Source: three-view drawing plus pictorial views. Frame: mm from the lowest corner of the part. Round coordinates to 2 decimals unless told otherwise and drop trailing zeros. Write each loop counter-clockwise with the first axis right and the second up, starting at its lowest first coordinate (ties: lowest second). Pieces come first, ordered by that corner, then holes. Notation, with made-up numbers: (2.25, 0.5) - (25.25, 0.5) arc R13 ccw to (25.25, 5.5) - close; hole circle Ø10 at (35.25, 76). An arc over 180 degrees is marked (long way). Write each question's results on one line, items separated by ' | '.
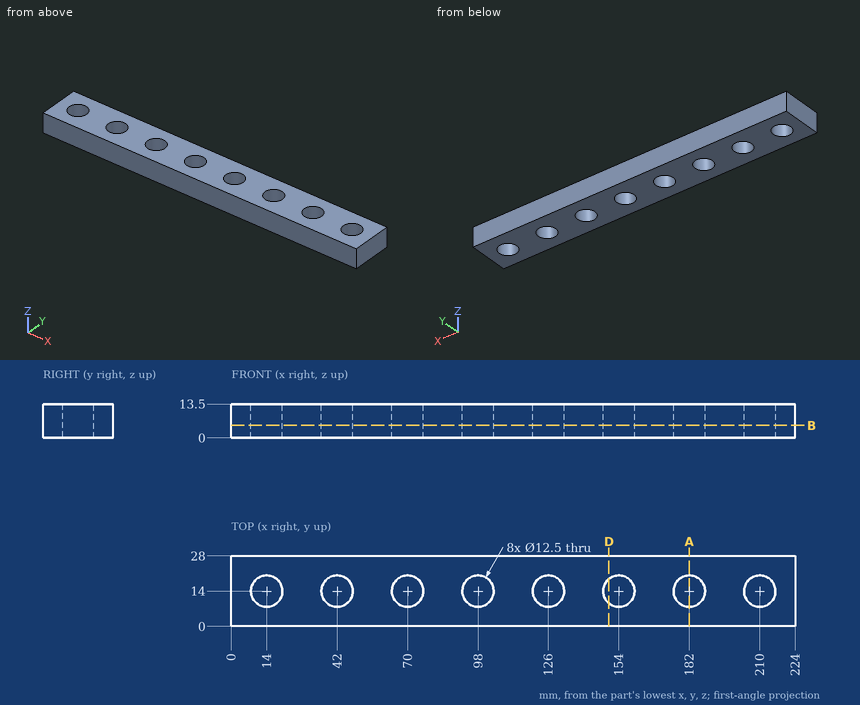
Q1. Section query D-D, the plane x = 150. Return loops of the section in (y, z), plus the area to 3 significant figures.
Answer block:
outline: (0, 0) - (9.2, 0) - (9.2, 13.5) - (0, 13.5) - close; (18.8, 0) - (28, 0) - (28, 13.5) - (18.8, 13.5) - close | area: 248 mm2
Q2. Pin query (flat end, axial travel): pin 1 (1.5 mm diameter, centred on y = 4.5, z = 5, fed in from -X); pin 2 (7.5 mm diameter, centred on x = 98, y = 14, fed in from -Z). Return the tip coordinate at first contact, or that it passes through.
Answer block:
pin 1: x = 0 | pin 2: through
Q3. Ray query, line 1 along Y through (x, z) = (42, 8); line 2 along Y through (x, z) = (96.5, 8.5). Return the intervals inside material, ascending.
Answer block:
line 1: 0 to 7.75, 20.25 to 28 | line 2: 0 to 7.93, 20.07 to 28
Q4. Section query B-B, the plane z = 5. Give the number of separate pieces and of enclosed holes in the cut face, plus the area to 3 significant figures.
Answer block:
separate pieces: 1 | enclosed holes: 8 | area: 5,290 mm2
Q5. Section query A-A, the plane x = 182. Return loops of the section in (y, z), plus the area to 3 significant figures.
Answer block:
outline: (0, 0) - (7.75, 0) - (7.75, 13.5) - (0, 13.5) - close; (20.25, 0) - (28, 0) - (28, 13.5) - (20.25, 13.5) - close | area: 209 mm2
